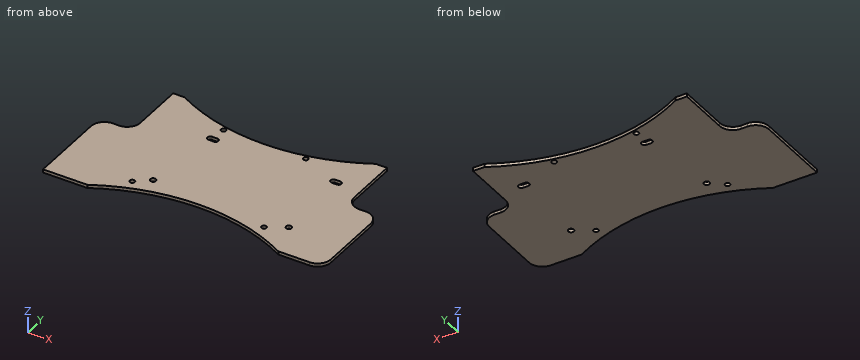
```python
from build123d import *

# Parameters (mm, degrees)
SKETCH2_R           = 1.5
SKETCH2_R_2         = 1.7
BOSS_EXTRUDE1_DEPTH = 2
FILLET4_R           = 8
SKETCH2_3_W         = 20
SKETCH2_3_H         = 55
BOSS_EXTRUDE2_DEPTH = 2
FILLET6_R           = 8
FILLET7_R           = 8


with BuildPart() as part:
    # Sketch2 → Boss-Extrude1 (new body)
    with BuildSketch(Plane.XY):
        with BuildLine():
            Line((65, 7.5), (65, 47.5))
            Line((65, 47.5), (58.094750193, 47.5))
            ThreePointArc((58.094750193, 47.5), (0, 32.5), (-58.094750193, 47.5))
            Line((-58.094750193, 47.5), (-65, 47.5))
            Line((-65, 47.5), (-65, 7.5))
            Line((-65, 7.5), (-85, 7.5))
            Line((-85, 7.5), (-85, -47.5))
            Line((-85, -47.5), (-58.094750193, -47.5))
            ThreePointArc((-58.094750193, -47.5), (0, -32.5), (58.094750193, -47.5))
            Line((58.094750193, -47.5), (65, -47.5))
            Line((65, -47.5), (65, 7.5))
        make_face()
        with Locations((-40, -32.5)):
            Circle(SKETCH2_R, mode=Mode.SUBTRACT)
        with Locations((-31.5, -25.8)):
            Circle(SKETCH2_R_2, mode=Mode.SUBTRACT)
        with Locations((40, -32.5)):
            Circle(SKETCH2_R, mode=Mode.SUBTRACT)
        with Locations((51, -25.8)):
            Circle(SKETCH2_R_2, mode=Mode.SUBTRACT)
        with BuildLine():
            ThreePointArc((-26.8, 20.76), (-28.5, 22.46), (-26.8, 24.16))
            Line((-26.8, 24.16), (-23.6, 24.16))
            ThreePointArc((-23.6, 24.16), (-21.9, 22.46), (-23.6, 20.76))
            Line((-23.6, 20.76), (-26.8, 20.76))
        make_face(mode=Mode.SUBTRACT)
        with Locations((-25, 32.5)):
            Circle(SKETCH2_R, mode=Mode.SUBTRACT)
        with BuildLine():
            ThreePointArc((48.015152789, 20.76), (46.315152789, 22.46), (48.015152789, 24.16))
            Line((48.015152789, 24.16), (51.215152789, 24.16))
            ThreePointArc((51.215152789, 24.16), (52.915152789, 22.46), (51.215152789, 20.76))
            Line((51.215152789, 20.76), (48.015152789, 20.76))
        make_face(mode=Mode.SUBTRACT)
        with Locations((25, 32.5)):
            Circle(SKETCH2_R, mode=Mode.SUBTRACT)
    extrude(amount=BOSS_EXTRUDE1_DEPTH)

    # Fillet4
    fillet4_edges = [part.edges().sort_by_distance(p)[0] for p in [
        (-85, 7.5, 1),
    ]]
    fillet(fillet4_edges, radius=FILLET4_R)

    # Sketch2<3> → Boss-Extrude2 (add)
    with BuildSketch(Plane.XY):
        with Locations((75, -20)):
            Rectangle(SKETCH2_3_W, SKETCH2_3_H)
    extrude(amount=BOSS_EXTRUDE2_DEPTH)

    # Fillet6
    fillet6_edges = [part.edges().sort_by_distance(p)[0] for p in [
        (85, -47.5, 1),
        (85, 7.5, 1),
        (65, 7.5, 1),
    ]]
    fillet(fillet6_edges, radius=FILLET6_R)

    # Fillet7
    fillet7_edges = [part.edges().sort_by_distance(p)[0] for p in [
        (-65, 7.5, 1),
    ]]
    fillet(fillet7_edges, radius=FILLET7_R)


solid = part.part
```
For this review, take the finished solid that the model builds, in its own axes (mm). Coordinates: 2 decimals unless noted, no trailing zeros. Write each loop counter-clockwise with the first axis right and the second up, starting at its lowest first coordinate (ties: lowest second). Pieces come first, ordered by that corner, then holes.
(1) Add section B-B on z = 1.7. Count the separate pieces of the cut face and the enclosed holes in it, then the cut area to 3 significant figures.
(2) For pin 1 Ø1 at (x, z) = (49.5, 1) entering from -Y; pin 2 Ø1 at (x, z) = (-41, 0.5) entering from +Y; pin 3 Ø1 at (x, z) = (-75, 1) entering from +Y, all flat-tipped, find the tip position at first contact; note any pin that passes through.
(3) Add section A-A on y = -25.8. Give the boundary of the cut face in (x, z), then the cut area to 3 significant figures.
(4) Add section D-D on y = 22.46. Give the boundary of the cut face in (x, z), then the cut area to 3 significant figures.
(5) Add section C-C on x = -31.5. Give the boundary of the cut face in (y, z).
(6) Wall thickness on probe 1 along Y at (x, z) = (51, 0.6); probe 2 along X at (y, z) = (15.5, 1.4); probe 3 along X at (y, z) = (-43, 1.1): over which ranges is each line inside the solid? List them lowest first.
Answer sheet:
1. separate pieces: 1
1. enclosed holes: 8
1. area: 12,100 mm2
2. pin 1: stops at y = -43.41
2. pin 2: stops at y = 39.9
2. pin 3: stops at y = 7.5
3. outline: (-85, 0) - (-33.2, 0) - (-33.2, 2) - (-85, 2) - close; (-29.8, 0) - (49.3, 0) - (49.3, 2) - (-29.8, 2) - close; (52.7, 0) - (85, 0) - (85, 2) - (52.7, 2) - close
3. area: 326 mm2
4. outline: (-65, 0) - (-28.5, 0) - (-28.5, 2) - (-65, 2) - close; (-21.9, 0) - (46.32, 0) - (46.32, 2) - (-21.9, 2) - close; (52.92, 0) - (65, 0) - (65, 2) - (52.92, 2) - close
4. area: 234 mm2
5. outline: (-36.71, 0) - (-27.5, 0) - (-27.5, 2) - (-36.71, 2) - close; (-24.1, 0) - (36.71, 0) - (36.71, 2) - (-24.1, 2) - close
6. probe 1: y = -43.88 to -27.5, -24.1 to 20.76, 24.16 to 43.88
6. probe 2: x = -65 to 65
6. probe 3: x = -85 to -49.09, 49.09 to 84.19
